Source: CAD feature listing. Evaluate the final solid. Frame: model axes, mm. A direction names the side the tool comes from. Coordinates: 2 decimals unless noted, no trailing zeros. Order: outer loops, then holes, each group sorted by start corner. A loop starts at its lowest first (then second) coordinate and runs counter-clockwise, first axis right, second up.
Item 1: Section B-B on y = 107. Return the cut outline in (x, z).
Item 2: Reachability of faces 1 (the flat face through (-89.228, 160, 5)), 2 (the flat face through (-138.228, 159, 5)), 3 (the flat face through (-138.228, -132, 5)) from +Z, -Z, +X, -X, +Y, -Y: full face, straight path, thin tool, end or side. Return the list, or none.
Item 3: Mould query, pull axis Y, two halves, no side actions, for faces 4 (the flat face through (-135, 173.678, 5)), 5 (the flat face through (-89.228, 242, 5)), 6 (the flat face through (-113, -149.475, 5)). Classes: released by +Y, released by -Y, zero draft, split by the parting line, or undercut.
Item 4: Section A-A on x = -85.5. Return the cut outline in (y, z), then the cut area to 3 significant figures.
Item 5: Ray query, line 1 (Y direction, x = -140, z = 2.25); line 2 (Y direction, x = -95, z = 8.25); line 3 (Y direction, x = -130, z = 4). Return the intervals inside material, ascending.
Item 6: Contact query for flat-ended pins moving along their axis: P1, Ø0.6, axis at y = -77, z = 3, coming from the +X side; P2, Ø3, axis at y = 232.5, z = 5, coming from the -X side. Output: stop coordinate, or through.
from build123d import *

# Parameters (mm, degrees)
EXTRUDE_1_DEPTH = 10


with BuildPart() as part:
    # Эскиз2 → Бобышка-Вытянуть1 (new body)
    with BuildSketch(Plane.XY):
        with BuildLine():
            Line((-89.227881483, -149.474789065), (-138.227881483, -149.474789065))
            Line((-138.227881483, -149.474789065), (-138.227881483, -114.872465065))
            Line((-138.227881483, -114.872465065), (-148.226492884, -114.839108588))
            Line((-148.226492884, -114.839108588), (-148.226492884, -104.839108588))
            Line((-148.226492884, -104.839108588), (-138.227881483, -104.672465065))
            Line((-138.227881483, -104.672465065), (-138.227881483, -76.322465065))
            Line((-138.227881483, -76.322465065), (-131.427881483, -76.322465065))
            Line((-131.427881483, -76.322465065), (-131.427881483, -77.522465065))
            Line((-131.427881483, -77.522465065), (-129.227881483, -77.522465065))
            Line((-129.227881483, -77.522465065), (-129.227881483, -76.322465065))
            Line((-129.227881483, -76.322465065), (-127.727881483, -76.322465065))
            Line((-127.727881483, -76.322465065), (-127.727881483, -73.222465065))
            Line((-127.727881483, -73.222465065), (-129.227881483, -73.222465065))
            Line((-129.227881483, -73.222465065), (-129.227881483, -72.022465065))
            Line((-129.227881483, -72.022465065), (-131.427881483, -72.022465065))
            Line((-131.427881483, -72.022465065), (-131.427881483, -73.222465065))
            Line((-131.427881483, -73.222465065), (-138.227881483, -73.222465065))
            Line((-138.227881483, -73.222465065), (-138.227881483, -44.872465065))
            Line((-138.227881483, -44.872465065), (-148.226492884, -44.839108588))
            Line((-148.226492884, -44.839108588), (-148.226492884, -34.839108588))
            Line((-148.226492884, -34.839108588), (-138.227881483, -34.672465065))
            Line((-138.227881483, -34.672465065), (-138.227881483, 135.127534935))
            Line((-138.227881483, 135.127534935), (-148.226492884, 135.160891412))
            Line((-148.226492884, 135.160891412), (-148.226492884, 145.160891412))
            Line((-148.226492884, 145.160891412), (-138.227881483, 145.327534935))
            Line((-138.227881483, 145.327534935), (-138.227881483, 173.677534935))
            Line((-138.227881483, 173.677534935), (-131.427881483, 173.677534935))
            Line((-131.427881483, 173.677534935), (-131.427881483, 172.477534935))
            Line((-131.427881483, 172.477534935), (-129.227881483, 172.477534935))
            Line((-129.227881483, 172.477534935), (-129.227881483, 173.677534935))
            Line((-129.227881483, 173.677534935), (-127.727881483, 173.677534935))
            Line((-127.727881483, 173.677534935), (-127.727881483, 176.777534935))
            Line((-127.727881483, 176.777534935), (-129.227881483, 176.777534935))
            Line((-129.227881483, 176.777534935), (-129.227881483, 177.977534935))
            Line((-129.227881483, 177.977534935), (-131.427881483, 177.977534935))
            Line((-131.427881483, 177.977534935), (-131.427881483, 176.777534935))
            Line((-131.427881483, 176.777534935), (-138.227881483, 176.777534935))
            Line((-138.227881483, 176.777534935), (-138.227881483, 186.777534935))
            Line((-138.227881483, 186.777534935), (-136.727881483, 186.777534935))
            ThreePointArc((-136.727881483, 186.777534935), (-135.667221312, 187.216874763), (-135.227881483, 188.277534935))
            Line((-135.227881483, 188.277534935), (-135.227881483, 190.277534935))
            ThreePointArc((-135.227881483, 190.277534935), (-135.667221312, 191.338195107), (-136.727881483, 191.777534935))
            Line((-136.727881483, 191.777534935), (-138.227881483, 191.777534935))
            Line((-138.227881483, 191.777534935), (-138.227881483, 205.127534935))
            Line((-138.227881483, 205.127534935), (-148.226492884, 205.160891412))
            Line((-148.226492884, 205.160891412), (-148.226492884, 215.160891412))
            Line((-148.226492884, 215.160891412), (-138.227881483, 215.327534935))
            Line((-138.227881483, 215.327534935), (-138.227881483, 268.427534935))
            Line((-138.227881483, 268.427534935), (-89.227881483, 268.427534935))
            Line((-89.227881483, 268.427534935), (-89.227881483, 215.327534935))
            Line((-89.227881483, 215.327534935), (-79.229270083, 215.160891412))
            Line((-79.229270083, 215.160891412), (-79.229270083, 205.160891412))
            Line((-79.229270083, 205.160891412), (-89.227881483, 205.127534935))
            Line((-89.227881483, 205.127534935), (-89.227881483, 176.777534935))
            Line((-89.227881483, 176.777534935), (-96.027881483, 176.777534935))
            Line((-96.027881483, 176.777534935), (-96.027881483, 177.977534935))
            Line((-96.027881483, 177.977534935), (-98.227881483, 177.977534935))
            Line((-98.227881483, 177.977534935), (-98.227881483, 176.777534935))
            Line((-98.227881483, 176.777534935), (-99.727881483, 176.777534935))
            Line((-99.727881483, 176.777534935), (-99.727881483, 173.677534935))
            Line((-99.727881483, 173.677534935), (-98.227881483, 173.677534935))
            Line((-98.227881483, 173.677534935), (-98.227881483, 172.477534935))
            Line((-98.227881483, 172.477534935), (-96.027881483, 172.477534935))
            Line((-96.027881483, 172.477534935), (-96.027881483, 173.677534935))
            Line((-96.027881483, 173.677534935), (-89.227881483, 173.677534935))
            Line((-89.227881483, 173.677534935), (-89.227881483, 145.327534935))
            Line((-89.227881483, 145.327534935), (-79.229270083, 145.160891412))
            Line((-79.229270083, 145.160891412), (-79.229270083, 135.160891412))
            Line((-79.229270083, 135.160891412), (-89.227881483, 135.127534935))
            Line((-89.227881483, 135.127534935), (-89.227881483, -34.672465065))
            Line((-89.227881483, -34.672465065), (-79.229270083, -34.839108588))
            Line((-79.229270083, -34.839108588), (-79.229270083, -44.839108588))
            Line((-79.229270083, -44.839108588), (-89.227881483, -44.872465065))
            Line((-89.227881483, -44.872465065), (-89.227881483, -73.222465065))
            Line((-89.227881483, -73.222465065), (-96.027881483, -73.222465065))
            Line((-96.027881483, -73.222465065), (-96.027881483, -72.022465065))
            Line((-96.027881483, -72.022465065), (-98.227881483, -72.022465065))
            Line((-98.227881483, -72.022465065), (-98.227881483, -73.222465065))
            Line((-98.227881483, -73.222465065), (-99.727881483, -73.222465065))
            Line((-99.727881483, -73.222465065), (-99.727881483, -76.322465065))
            Line((-99.727881483, -76.322465065), (-98.227881483, -76.322465065))
            Line((-98.227881483, -76.322465065), (-98.227881483, -77.522465065))
            Line((-98.227881483, -77.522465065), (-96.027881483, -77.522465065))
            Line((-96.027881483, -77.522465065), (-96.027881483, -76.322465065))
            Line((-96.027881483, -76.322465065), (-89.227881483, -76.322465065))
            Line((-89.227881483, -76.322465065), (-89.227881483, -104.672465065))
            Line((-89.227881483, -104.672465065), (-79.229270083, -104.839108588))
            Line((-79.229270083, -104.839108588), (-79.229270083, -114.839108588))
            Line((-79.229270083, -114.839108588), (-89.227881483, -114.872465065))
            Line((-89.227881483, -114.872465065), (-89.227881483, -149.474789065))
        make_face()
    extrude(amount=EXTRUDE_1_DEPTH)


solid = part.part
Answer list:
1. outline: (-138.23, 0) - (-89.23, 0) - (-89.23, 10) - (-138.23, 10) - close
2. face 1: +Z, -Z, +X
2. face 2: +Z, -Z, -X
2. face 3: +Z, -Z, -X, -Y
3. face 4: undercut
3. face 5: zero draft
3. face 6: released by -Y
4. outline: (-114.86, 0) - (-104.73, 0) - (-104.73, 10) - (-114.86, 10) - close; (-44.86, 0) - (-34.73, 0) - (-34.73, 10) - (-44.86, 10) - close; (135.14, 0) - (145.27, 0) - (145.27, 10) - (135.14, 10) - close; (205.14, 0) - (215.27, 0) - (215.27, 10) - (205.14, 10) - close
4. area: 405 mm2
5. line 1: y = -114.87 to -104.7, -44.87 to -34.7, 135.13 to 145.3, 205.13 to 215.3
5. line 2: y = -149.47 to -76.32, -73.22 to 173.68, 176.78 to 268.43
5. line 3: y = -149.47 to -77.52, -72.02 to 172.48, 177.98 to 268.43
6. P1: stops at x = -89.23
6. P2: stops at x = -138.23
